```python
from build123d import *

# Parameters (mm, degrees)
PAD_DEPTH    = 0.6
SKETCH001_W  = 3
SKETCH001_H  = 1
PAD001_DEPTH = 3


with BuildPart() as part:
    # Sketch → Pad (new body)
    with BuildSketch(Plane.XY):
        Polygon((-0.75, 1.5), (-1.5, 1.5), (-1.5, -1.5), (1.5, -1.5), (1.5, 1.5), (0.75, 1.5), (3.264603, 2.4375), (-1.764603, 4.3125), (3.264603, 6.1875), (-1.764603, 8.0625), (0.75, 9), (1.5, 9), (1.5, 10), (-1.5, 10), (-1.5, 9), (-0.75, 9), (-3.264603, 8.0625), (1.764603, 6.1875), (-3.264603, 4.3125), (1.764603, 2.4375), align=None)
    extrude(amount=PAD_DEPTH)

    # Sketch001 → Pad001 (new body)
    with BuildSketch(Plane.XY.offset(0.6)):
        with Locations((0, 9.5)):
            Rectangle(SKETCH001_W, SKETCH001_H)
    extrude(amount=PAD001_DEPTH)


solid = part.part
```
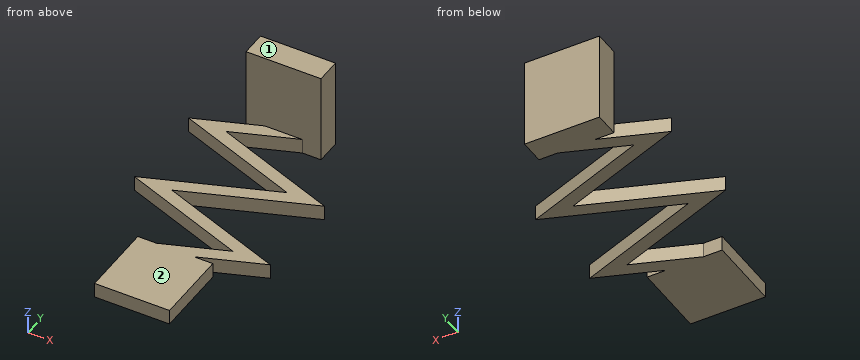
Check sheet for the modelled part. Datum: model origin and axes. Units: mm. Face numbers are marked on the shaded views. A direction names the side the tool comes from. Coordinates: 2 decimals unless noted, no trailing zeros. Write each loop counter-clockwise with the first axis right and the second up, starting at its lowest first coordinate (ties: lowest second). Pieces come first, ordered by that corner, then holes. Notation, with made-up numbers: (-17.75, -17) -> (39.25, -17) arc R20 ccw to (39.25, -1) -> close; hole circle Ø1 at (13, -36). An arc over 180 degrees is marked (long way). Use a Markdown table: item, result.
1. Sectioned sample at C-C (y = -0.5). Enter the section's corners in (x, z), plus the area to 3 significant figures.
Reported:
| item | result |
|---|---|
| outline | (-1.5, 0) -> (1.5, 0) -> (1.5, 0.6) -> (-1.5, 0.6) -> close |
| area | 1.80 mm2 |
2. Go/stop test with flat-tipped pins: pin 1 Ø1 at (y, z) = (1.5, 2.5) entering from +X; pin 2 Ø0.8 at (y, z) = (9.5, 1) entering from +X; pin 3 Ø2 at (x, y) = (0, 5) entering from -Z. Record where each tip stops, or that it passes through.
Reported:
| item | result |
|---|---|
| pin 1 | passes through |
| pin 2 | stops at x = 1.5 |
| pin 3 | stops at z = 0 |
3. Scan lines: line 1 along Z through (x, y) = (-0.75, 8.5); line 2 along Y through (x, z) = (-1.25, 1.4); line 3 along X through (y, z) = (-1, 0.2). Record each from-to range of solid material in increasing order.
Reported:
| item | result |
|---|---|
| line 1 | z = 0 to 0.6 |
| line 2 | y = 9 to 10 |
| line 3 | x = -1.5 to 1.5 |
4. Sectioned sample at D-D (z = 3.45). Enter the section's corners in (x, y).
Reported:
| item | result |
|---|---|
| outline | (-1.5, 9) -> (1.5, 9) -> (1.5, 10) -> (-1.5, 10) -> close |
5. Tool access check on the marked faces 1 and 2. Record the directions out of +Z, -Z, +X, -X, +Y, -Y that give a thin tool (end or side, any length) a straight path to the whole face; none if there is none.
Reported:
| item | result |
|---|---|
| face 1 | +Z, +X, -X, +Y, -Y |
| face 2 | +Z, +X, -X, -Y |
6. Sectioned sample at B-B (x = -2.5). Enter the section's corners in (y, z).
Reported:
| item | result |
|---|---|
| outline | (4.03, 0) -> (4.6, 0) -> (4.6, 0.6) -> (4.03, 0.6) -> close; (7.78, 0) -> (8.35, 0) -> (8.35, 0.6) -> (7.78, 0.6) -> close |
7. Sectioned sample at A-A (x = 0.5). Enter the section's corners in (y, z).
Reported:
| item | result |
|---|---|
| outline | (-1.5, 0) -> (1.97, 0) -> (1.97, 0.6) -> (-1.5, 0.6) -> close; (2.91, 0) -> (3.47, 0) -> (3.47, 0.6) -> (2.91, 0.6) -> close; (5.16, 0) -> (5.72, 0) -> (5.72, 0.6) -> (5.16, 0.6) -> close; (6.66, 0) -> (7.22, 0) -> (7.22, 0.6) -> (6.66, 0.6) -> close; (8.91, 0) -> (10, 0) -> (10, 3.6) -> (9, 3.6) -> (9, 0.6) -> (8.91, 0.6) -> close |
